Input: dimensioned drawing with shaded views. Units: mm. Origin: part minimum x, y, z. Round coordinates to 2 decimals unless told otherwise and drop trailing zeros. Order: outer loops, then holes, each group sorted by start corner. A loop starts at its lowest first (then second) coordinate and runs counter-clockwise, first axis right, second up. Notation, with made-up numbers: (68.5, -21) - (107.5, -21) arc R17 ccw to (107.5, -16) - close; hole circle Ø6 at (21.5, 56). An arc over 180 degrees is marked (long way). Return JSON: item names as keys, results as strings. Group by question number.
1) Section B-B, the plane x = 28. Return loops of the section in (y, z).
2) Ray query, line 1 (X direction, y = 2.15, z = 8.5); line 2 (X direction, y = 3.1, z = 14) (3 decimals); line 3 (Z direction, x = 83.5, y = 4.15). Return the intervals inside material, ascending. Write a range as from..to.
3) Section C-C, the plane y = 2.8. Give the number of separate pieces and of enclosed holes in the cut face, plus the area to 3 significant figures.
4) Section A-A, the plane z = 28. Return loops of the section in (x, y) (3 decimals), plus the area to 3 significant figures.
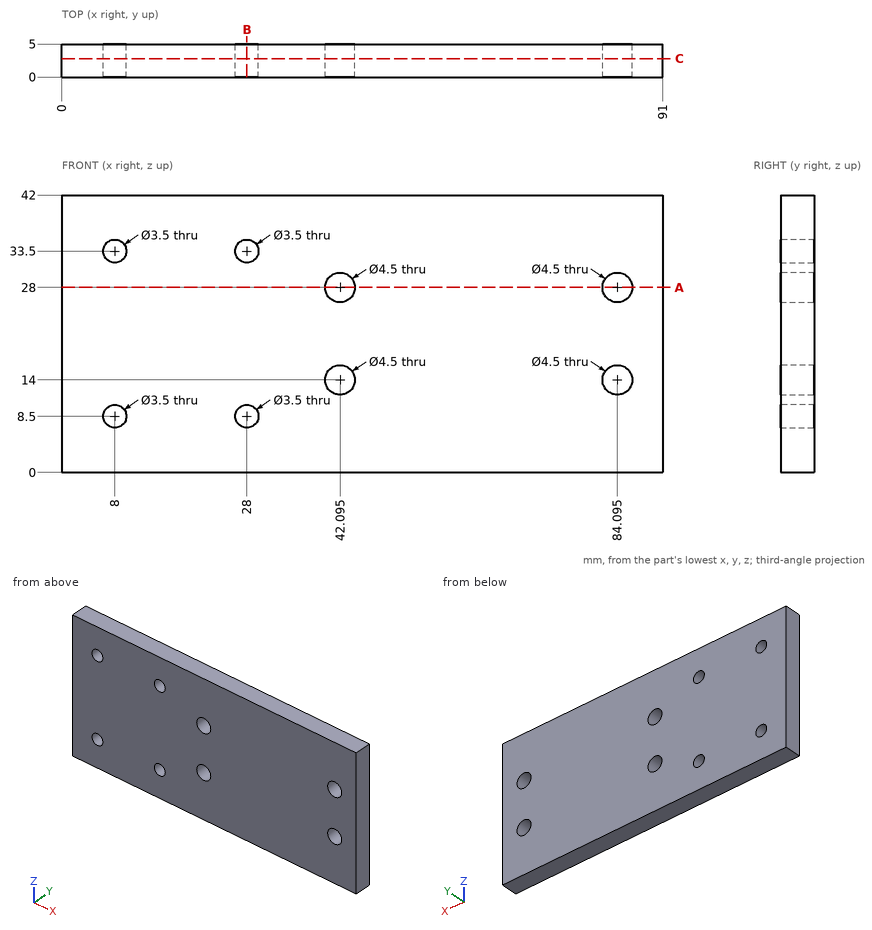
Geometry check:
{
 "1": {"outline": "(0, 0) - (5, 0) - (5, 6.75) - (0, 6.75) - close; (0, 10.25) - (5, 10.25) - (5, 31.75) - (0, 31.75) - close; (0, 35.25) - (5, 35.25) - (5, 42) - (0, 42) - close"},
 "2": {"line 1": "0..6.25, 9.75..26.25, 29.75..91", "line 2": "0..39.845, 44.345..81.845, 86.345..91", "line 3": "0..11.83, 16.17..25.83, 30.17..42"},
 "3": {"separate pieces": "1", "enclosed holes": "8", "area": "3,720 mm2"},
 "4": {"outline": "(0, 0) - (39.845, 0) - (39.845, 5) - (0, 5) - close; (44.345, 0) - (81.845, 0) - (81.845, 5) - (44.345, 5) - close; (86.345, 0) - (91, 0) - (91, 5) - (86.345, 5) - close", "area": "410 mm2"}
}
